Source: CAD feature listing. Evaluate the final solid. Frame: model axes, mm. Round coordinates to 2 decimals unless told otherwise and drop trailing zeros. Loops run counter-clockwise (first coordinate to the right, second up) from the corner with the lowest first, then second, coordinate; pieces in that order, holes last. Notation, with made-up numbers: M 87,58.25 L 103,58.25 A25 cw 103,79.25 Z; hole C -15.5,-31.75 d3. An arc over 180 degrees is marked long. One line per item, written item: value.
from build123d import *

# Parameters (mm, degrees)
SKETCH1_W           = 45
SKETCH1_H           = 45
BOSS_EXTRUDE1_DEPTH = 50
SKETCH2_R           = 4.15
CUT_EXTRUDE1_DEPTH  = 30
SKETCH3_R           = 4.15
CUT_EXTRUDE2_DEPTH  = 30
CHAMFER1_SIZE       = 3


with BuildPart() as part:
    # Sketch1 → Boss-Extrude1 (new body)
    with BuildSketch(Plane(origin=(0, 0, 0), x_dir=(1, 0, 0), z_dir=(0, 1, 0))):
        Rectangle(SKETCH1_W, SKETCH1_H)
    extrude(amount=BOSS_EXTRUDE1_DEPTH)

    # Sketch2 → Cut-Extrude1 (cut)
    with BuildSketch(Plane(origin=(0, 0, -22.5), x_dir=(-1, 0, 0), z_dir=(0, 0, -1))):
        with Locations((0, 12.5)):
            Circle(SKETCH2_R)
    extrude(amount=-CUT_EXTRUDE1_DEPTH, mode=Mode.SUBTRACT)

    # Sketch3 → Cut-Extrude2 (cut)
    with BuildSketch(Plane.ZY.offset(22.5)):
        with Locations((0, 37.5)):
            Circle(SKETCH3_R)
    extrude(amount=-CUT_EXTRUDE2_DEPTH, mode=Mode.SUBTRACT)

    # Chamfer1
    chamfer1_edges = [part.edges().sort_by_distance(p)[0] for p in [
        (-22.5, 50, 0),
        (0, 50, 22.5),
        (22.5, 50, 0),
        (0, 0, 22.5),
        (-22.5, 0, 0),
        (0, 0, -22.5),
        (22.5, 0, 0),
        (22.5, 25, 22.5),
        (-22.5, 25, 22.5),
        (-22.5, 25, -22.5),
        (22.5, 25, -22.5),
        (0, 50, -22.5),
    ]]
    chamfer(chamfer1_edges, length=CHAMFER1_SIZE)


solid = part.part
1. Section query C-C (y = 12.5). Return the cut outline in (x, z), and give its area (3 significant figures).
Report:
outline: M -22.5,-19.5 L -19.5,-22.5 L -4.15,-22.5 L -4.15,7.5 L 4.15,7.5 L 4.15,-22.5 L 19.5,-22.5 L 22.5,-19.5 L 22.5,19.5 L 19.5,22.5 L -19.5,22.5 L -22.5,19.5 Z
area: 1,760 mm2
2. Pin query (flat end, axial travel): pin 1 (7.5 mm diameter, centred on y = 37.5, z = 0, fed in from -X). Return the tip coordinate at first contact, or that it passes through.
Report:
pin 1: stops at x = 7.5
3. Pull-direction query (Z, two-part tool) for faces 1 (the face through (-7.71, 41.615, -0.54)), 2 (the face through (21, 25, -21)), 3 (the face through (21, 48, 20)); classes: released by +Z, released by -Z, zero draft, split by the parting line, or undercut.
Report:
face 1: undercut
face 2: released by -Z
face 3: released by +Z
4. Section query B-B (x = -14). Return the cut outline in (y, z).
Report:
outline: M 0,-19.5 L 3,-22.5 L 47,-22.5 L 50,-19.5 L 50,19.5 L 47,22.5 L 3,22.5 L 0,19.5 Z; hole C 37.5,0 d8.3
5. Section query A-A (z = 0). Return the cut outline in (x, y).
Report:
outline: M -22.5,3 L -19.5,0 L 19.5,0 L 22.5,3 L 22.5,47 L 19.5,50 L -19.5,50 L -22.5,47 L -22.5,41.65 L 7.5,41.65 L 7.5,33.35 L -22.5,33.35 Z; hole C 0,12.5 d8.3
6. Section query D-D (z = -5). Return the cut outline in (x, y), and give its area (3 significant figures).
Report:
outline: M -22.5,3 L -19.5,0 L 19.5,0 L 22.5,3 L 22.5,47 L 19.5,50 L -19.5,50 L -22.5,47 Z; hole C 0,12.5 d8.3
area: 2,180 mm2
7. Ray query, line 1 (Y direction, x = -3, z = 0); line 2 (Y direction, x = 0, z = 0); line 3 (Y direction, x = 0, z = -13.25). Return the intervals inside material, ascending. Write a range as [from, to].
Report:
line 1: y = [0, 9.63], [15.37, 33.35], [41.65, 50]
line 2: y = [0, 8.35], [16.65, 33.35], [41.65, 50]
line 3: y = [0, 8.35], [16.65, 50]
